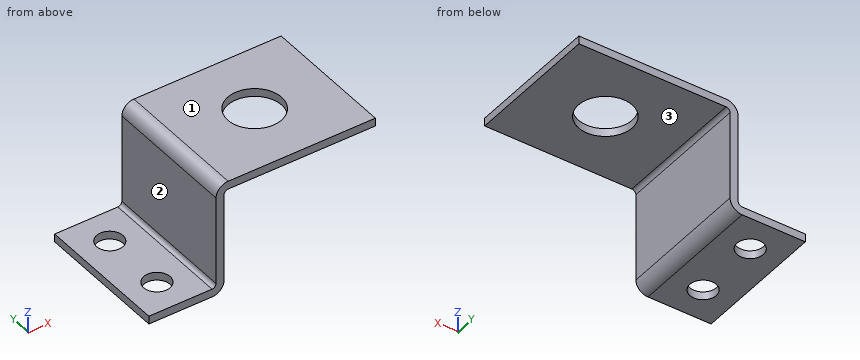
```python
from build123d import *

# Parameters (mm, degrees)
SKETCH5_W                    = 12.7
SKETCH5_H                    = 25.4
BASE_FLANGE1_DEPTH           = 1.524
EDGE_FLANGE1_STRIP_W         = 7.62
EDGE_FLANGE1_STRIP_H         = 1.524
EDGE_FLANGE1_STRIP_CUT_DEPTH = 25.4
EDGE_FLANGE1_DEPTH           = 25.4
EDGE_FLANGE2_STRIP_W         = 7.62
EDGE_FLANGE2_STRIP_H         = 1.524
EDGE_FLANGE2_STRIP_CUT_DEPTH = 25.4
EDGE_FLANGE2_DEPTH           = 25.4
CUT_EXTRUDE1_REACH           = 56.123
SKETCH16_R                   = 5.08
F_10_CLEARANCE_HOLE2_D       = 4.9784


# Sheet-metal steps are written as plain solids
with BuildPart() as part:
    # Sketch5 → Base-Flange1 (new body)
    with BuildSketch(Plane.XY):
        with Locations((6.35, 12.7)):
            Rectangle(SKETCH5_W, SKETCH5_H)
    extrude(amount=-BASE_FLANGE1_DEPTH)

    # Edge-Flange1 strip (across the edge) → Edge-Flange1 strip cut (cut)
    with BuildSketch(Plane(origin=(12.7, 0, 0), x_dir=(-1, 0, 0), z_dir=(0, 1, 0))):
        with Locations((-3.048, -0.762)):
            Rectangle(EDGE_FLANGE1_STRIP_W, EDGE_FLANGE1_STRIP_H)
    extrude(amount=EDGE_FLANGE1_STRIP_CUT_DEPTH, mode=Mode.SUBTRACT)

    # Edge-Flange1 section (across the edge) → Edge-Flange1 (add)
    with BuildSketch(Plane(origin=(12.7, 0, 0), x_dir=(-1, 0, 0), z_dir=(0, 1, 0))):
        with BuildLine():
            Line((-1.524, 0.762), (-1.524, 18.22041314))
            Line((-1.524, 18.22041314), (0, 18.22041314))
            Line((0, 18.22041314), (0, 0.762))
            ThreePointArc((0, 0.762), (0.223184633, 0.223184633), (0.762, 0))
            Line((0.762, 0), (0.762, -1.524))
            ThreePointArc((0.762, -1.524), (-0.854446102, -0.854446102), (-1.524, 0.762))
        make_face()
    extrude(amount=EDGE_FLANGE1_DEPTH)

    # Edge-Flange2 strip (across the edge) → Edge-Flange2 strip cut (cut)
    with BuildSketch(Plane(origin=(14.224, 25.4, 18.22041314), x_dir=(0, 0, -1), z_dir=(0, -1, 0))):
        with Locations((-3.048, -0.762)):
            Rectangle(EDGE_FLANGE2_STRIP_W, EDGE_FLANGE2_STRIP_H)
    extrude(amount=EDGE_FLANGE2_STRIP_CUT_DEPTH, mode=Mode.SUBTRACT)

    # Edge-Flange2 section (across the edge) → Edge-Flange2 (add)
    with BuildSketch(Plane(origin=(14.224, 25.4, 18.22041314), x_dir=(0, 0, -1), z_dir=(0, -1, 0))):
        with BuildLine():
            Line((-1.524, 0.762), (-1.524, 28.575))
            Line((-1.524, 28.575), (0, 28.575))
            Line((0, 28.575), (0, 0.762))
            ThreePointArc((0, 0.762), (0.223184633, 0.223184633), (0.762, 0))
            Line((0.762, 0), (0.762, -1.524))
            ThreePointArc((0.762, -1.524), (-0.854446102, -0.854446102), (-1.524, 0.762))
        make_face()
    extrude(amount=EDGE_FLANGE2_DEPTH)

    # Sketch16 → Cut-Extrude1 (cut, up to next)
    with BuildSketch(Plane.XY.offset(19.74441314), mode=Mode.PRIVATE) as cut_extrude1_sk1:
        with Locations((28.8925, 12.7)):
            Circle(SKETCH16_R)
    cut_extrude1_tool1 = extrude(cut_extrude1_sk1.sketch, amount=-CUT_EXTRUDE1_REACH, mode=Mode.PRIVATE) & part.part
    add(cut_extrude1_tool1.solids().sort_by_distance((28.8925, 12.7, 19.744413))[0], mode=Mode.SUBTRACT)

    # #10 Clearance Hole2 (through all)
    with Locations(Plane.XY):
        with Locations((5.969, 19.05), (5.969, 6.35)):
            Hole(F_10_CLEARANCE_HOLE2_D / 2)


solid = part.part
```
Work out the finished part from the listing and answer in its coordinate system (mm). Face numbers are marked on the shaded views. A direction names the side the tool comes from. Round coordinates to 2 decimals unless told otherwise and drop trailing zeros. Write each loop counter-clockwise with the first axis right and the second up, starting at its lowest first coordinate (ties: lowest second). Pieces come first, ordered by that corner, then holes. Notation, with made-up numbers: (3, 81) - (23, 81) arc R30 ccw to (23, 110) - close; hole circle Ø5 at (-32, 14). An arc over 180 degrees is marked (long way). Return JSON: item names as keys, results as strings. Group by question number.
Q1. The part is cut by section C-C on y = 12.7. Write down the section's boundary in (x, z).
Q2. For the marked faces 1, 2 and 3, determine the directions among +Z, -Z, +X, -X, +Y, -Y from which every point of the face is accessible in a straight line to the end or side of a thin tool.
Q3. The part is cut by section B-B on x = 25. Write down the section's boundary in (y, z).
Q4. Each of these flat-tipped pins is pushed along its axis until it touches: pin 1 Ø6.5 at (x, y) = (5.969, 6.35) entering from -Z; pin 2 Ø8 at (x, y) = (28.89, 12.7) entering from -Z; pin 3 Ø2 at (y, z) = (9.5, 13.5) entering from +X; pin 4 Ø8 at (x, y) = (5.969, 19.05) entering from +Z. Where does it stop, or does it pass through?
Q5. The part is cut by section D-D on z = 10.25. Write down the section's boundary in (x, y).
Q6. Find the intervals of material crossed by L1, parallel to Z at x = 19.5, y = 19.25; L2, parallel to X at y = 13.75, z = 1; L3, parallel to Z at x = 10, y = 19, in increasing order.
Q7. The part is cut by section A-A on y = 19.05. Write down the section's boundary in (x, z), then the cut area to 3 significant figures.
Solved:
{
 "1": {"outline": "(0, -1.52) - (11.94, -1.52) arc R2.29 ccw to (14.22, 0.76) - (14.22, 17.46) arc R0.76 cw to (14.99, 18.22) - (23.81, 18.22) - (23.81, 19.74) - (14.99, 19.74) arc R2.29 ccw to (12.7, 17.46) - (12.7, 0.76) arc R0.76 cw to (11.94, 0) - (0, 0) - close; (33.97, 18.22) - (42.8, 18.22) - (42.8, 19.74) - (33.97, 19.74) - close"},
 "2": {"face 1": "+Z, +X, -X, +Y, -Y", "face 2": "+Z, -X, +Y, -Y", "face 3": "-Z, +X, +Y, -Y"},
 "3": {"outline": "(0, 18.22) - (9.44, 18.22) - (9.44, 19.74) - (0, 19.74) - close; (15.96, 18.22) - (25.4, 18.22) - (25.4, 19.74) - (15.96, 19.74) - close"},
 "4": {"pin 1": "z = -1.52", "pin 2": "through", "pin 3": "x = 14.22", "pin 4": "z = 0"},
 "5": {"outline": "(12.7, 0) - (14.22, 0) - (14.22, 25.4) - (12.7, 25.4) - close"},
 "6": {"L1": "18.22 to 19.74", "L2": "12.7 to 14.22", "L3": "-1.52 to 0"},
 "7": {"outline": "(0, -1.52) - (3.48, -1.52) - (3.48, 0) - (0, 0) - close; (8.46, -1.52) - (11.94, -1.52) arc R2.29 ccw to (14.22, 0.76) - (14.22, 17.46) arc R0.76 cw to (14.99, 18.22) - (42.8, 18.22) - (42.8, 19.74) - (14.99, 19.74) arc R2.29 ccw to (12.7, 17.46) - (12.7, 0.76) arc R0.76 cw to (11.94, 0) - (8.46, 0) - close", "area": "85.7 mm²"}
}
